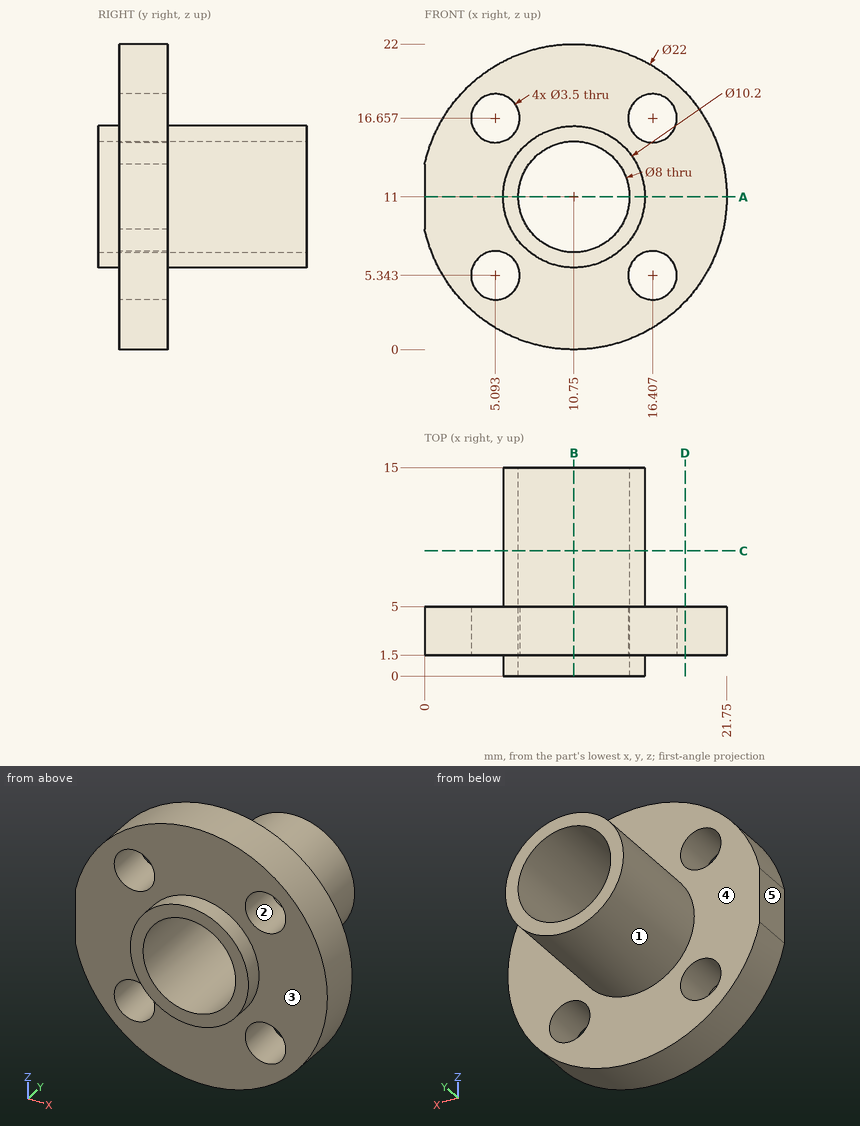
Check sheet for the drawn part. Datum: minimum x, y, z corner. Units: mm. A direction names the side the tool comes from. Round coordinates to 2 decimals unless told otherwise and drop trailing zeros. Order: outer loops, then holes, each group sorted by start corner. A loop starts at its lowest first (then second) coordinate and runs counter-clockwise, first axis right, second up. Notation, with made-up numbers: M 66,2 L 76,2 A9 ccw 76,11 Z; hole C 88.25,65.25 d7. An arc over 180 degrees is marked long. Answer in a Markdown table with one row per item.
(1) Material ranges on line 1 along Z through (x, y) = (10.75, 7); line 2 along Y through (x, z) = (16.25, 8); line 3 along X through (y, z) = (4, 14.25), recorded low to high. Write a range as from..to.
Findings:
| item | result |
|---|---|
| line 1 | z = 5.9..7, 15..16.1 |
| line 2 | y = 1.5..5 |
| line 3 | x = 0.24..8.42, 13.08..21.26 |
(2) Set-up check for the marked faces 4 and 5: record each of +Z, -Z, +X, -X, +Y, -Y from which the full face is reachable in a straight line by a thin tool's end or side.
Findings:
| item | result |
|---|---|
| face 4 | +Y |
| face 5 | +Z, -Z, -X, +Y, -Y |
(3) Section check C-C on y = 9. Record the boundary of the cut face in (x, z).
Findings:
| item | result |
|---|---|
| outline | C 10.75,11 d10.2; hole C 10.75,11 d8 |
(4) Gauge pin test, flat ends, axial feed: pin 1 (1.5 mm diameter, centred on y = 9, z = 11, fed in from +X); pin 2 (3 mm diameter, centred on x = 13, y = 3.5, fed in from -Z); pin 3 (5.5 mm diameter, centred on x = 16.41, z = 16.66, fed in from -Y). Record the tip position at first contact, or that the pin passes through.
Findings:
| item | result |
|---|---|
| pin 1 | stops at x = 15.85 |
| pin 2 | stops at z = 0.03 |
| pin 3 | stops at y = 1.5 |
(5) Draft check along X on the marked faces 1, 2 and 3. Enter one of: +X half, -X half, draft (parallel to the pull), parting line (faces both ways), or undercut.
Findings:
| item | result |
|---|---|
| face 1 | parting line |
| face 2 | undercut |
| face 3 | draft |
(6) Section check A-A on z = 11. Record the boundary of the cut face in (x, y).
Findings:
| item | result |
|---|---|
| outline | M 0,1.5 L 5.65,1.5 L 5.65,0 L 6.75,0 L 6.75,15 L 5.65,15 L 5.65,5 L 0,5 Z; M 14.75,0 L 15.85,0 L 15.85,1.5 L 21.75,1.5 L 21.75,5 L 15.85,5 L 15.85,15 L 14.75,15 Z |
(7) Section check D-D on x = 18.75. Record the boundary of the cut face in (y, z).
Findings:
| item | result |
|---|---|
| outline | M 1.5,3.45 L 5,3.45 L 5,18.55 L 1.5,18.55 Z |
(8) Section check B-B on x = 10.75. Record the boundary of the cut face in (y, z).
Findings:
| item | result |
|---|---|
| outline | M 0,5.9 L 1.5,5.9 L 1.5,0 L 5,0 L 5,5.9 L 15,5.9 L 15,7 L 0,7 Z; M 0,15 L 15,15 L 15,16.1 L 5,16.1 L 5,22 L 1.5,22 L 1.5,16.1 L 0,16.1 Z |
